Check sheet for the modelled part. Datum: model origin and axes. Units: mm. A direction names the side the tool comes from. Give positions to 0.01 mm unless a question says otherwise; leave off trailing zeros. Write each loop counter-clockwise with the first axis right and the second up, starting at its lowest first coordinate (ties: lowest second). Pieces come first, ordered by that corner, then holes. Notation, with made-up numbers: (89, 56.25) -> (114, 56.25) arc R20 cw to (114, 85.25) -> close; hole circle Ø10 at (-35, 72). An arc over 180 degrees is marked (long way). Answer as a JSON object with one key per item and string values.
from build123d import *

# Parameters (mm, degrees)
SKETCH1_R           = 1.8
SKETCH1_R_2         = 1
BOSS_EXTRUDE1_DEPTH = 11.5
SKETCH2_R           = 2
BOSS_EXTRUDE2_DEPTH = 0.5
CHAMFER1_SIZE       = 0.25
CHAMFER1_SIZE2      = 0.433012702
FILLET1_R           = 0.3


with BuildPart() as part:
    # Sketch1 → Boss-Extrude1 (new body)
    with BuildSketch(Plane(origin=(0, 0, 0), x_dir=(1, 0, 0), z_dir=(0, 1, 0))):
        with Locations(Location((0, 0, 0), (0, 0, 270))):
            Circle(SKETCH1_R)
        with Locations(Location((0, 0, 0), (0, 0, 270))):
            Circle(SKETCH1_R_2, mode=Mode.SUBTRACT)
    extrude(amount=BOSS_EXTRUDE1_DEPTH)

    # Sketch2 → Boss-Extrude2 (add)
    with BuildSketch(Plane(origin=(0, 11.5, 0), x_dir=(1, 0, 0), z_dir=(0, 1, 0))):
        with Locations(Location((0, 0, 0), (0, 0, 270))):
            Circle(SKETCH2_R)
    extrude(amount=BOSS_EXTRUDE2_DEPTH)

    # Chamfer1
    chamfer1_edges = [part.edges().sort_by_distance(p)[0] for p in [
        (0, 0, -1.8),
    ]]
    chamfer1_side = [part.faces().sort_by_distance(p)[0] for p in [
        (0, 0, -1.749088312),
    ]]
    chamfer(chamfer1_edges, length=CHAMFER1_SIZE, length2=CHAMFER1_SIZE2, reference=chamfer1_side[0])

    # Fillet1
    fillet1_edges = [part.edges().sort_by_distance(p)[0] for p in [
        (0, 0.433012702, -1.8),
    ]]
    fillet(fillet1_edges, radius=FILLET1_R)


solid = part.part
1. Mould release check, pull along Z, two halves, no side actions. Record for faces 1 (the face through (0, 12, 0)), 2 (the face through (-1, 6, 0)), 3 (the face through (-1.597, 5.93, 0.831)): released by +Z, released by -Z, zero draft, split by the parting line, or undercut.
Determined:
{"face 1": "zero draft", "face 2": "undercut", "face 3": "split by the parting line"}
2. Access from +Z, -Z, +X, -X, +Y, -Y to the whole of each face (thin tool, end or side, straight path). Record for faces 4 (the face through (0, 11.5, 0)), 5 (the face through (-1.952, 11.746, -0.434)).
Determined:
{"face 4": "-Y", "face 5": "+Y, -Y"}
3. Go/stop test with a flat-tipped pin: P1, Ø2, axis at x = 1, y = 2, coming from the +Z side. Record where the tip stops, or that it passes through.
Determined:
{"P1": "z = 1.8"}
4. Scan lines: L1, parallel to X at y = 3, z = 0; L2, parallel to Y at x = 0.3, z = -0.55. Record each from-to range of solid material in increasing order. Write a range as [from, to].
Determined:
{"L1": "[-1.8, -1], [1, 1.8]", "L2": "[11.5, 12]"}
5. Sectioned sample at A-A, the plane y = 4.5. Enter the section's corners in (x, z).
Determined:
{"outline": "circle Ø3.6 at (0, 0); hole circle Ø2 at (0, 0)"}
